from build123d import *

# Parameters (mm, degrees)
SKETCH_1_W                  = 80
SKETCH_1_H                  = 60
EXTRUDE_1_DEPTH             = 20
SKETCH_2_W                  = 72
SKETCH_2_H                  = 52
CUT_EXTRUDE_1_DEPTH         = 15
CUT_EXTRUDE_2_DEPTH         = 53.201532545
SKETCH_4_R                  = 1.6
CUT_EXTRUDE_3_DEPTH         = 53.201532545
PATTERN_LINEAR_1_COUNT      = 2
PATTERN_LINEAR_1_PITCH      = 60
PATTERN_LINEAR_1_COUNT_DIR2 = 2
PATTERN_LINEAR_1_PITCH_DIR2 = 40
FILLET_1_R                  = 5
SKETCH_5_W                  = 72
SKETCH_5_H                  = 52
CUT_EXTRUDE_4_DEPTH         = 1.5
SKETCH_6_W                  = 40
SKETCH_6_H                  = 8
CUT_EXTRUDE_7_DEPTH         = 85.118963379
SKETCH_7_W                  = 36
SKETCH_7_H                  = 6
CUT_EXTRUDE_8_DEPTH         = 85.118963379
SKETCH_8_W                  = 74
SKETCH_8_H                  = 54
CUT_EXTRUDE_9_DEPTH         = 1.5
SKETCH_9_W                  = 74
SKETCH_9_H                  = 54
CUT_EXTRUDE_10_DEPTH        = 1.5


with BuildPart() as part:
    # 草图1 → 凸台-拉伸1 (new body)
    with BuildSketch(Plane(origin=(0, 0, 0), x_dir=(1, 0, 0), z_dir=(0, 1, 0))):
        Rectangle(SKETCH_1_W, SKETCH_1_H)
    extrude(amount=EXTRUDE_1_DEPTH)

    # 草图2 → 切除-拉伸1 (cut)
    with BuildSketch(Plane(origin=(0, 20, 0), x_dir=(1, 0, 0), z_dir=(0, 1, 0))):
        Rectangle(SKETCH_2_W, SKETCH_2_H)
    extrude(amount=-CUT_EXTRUDE_1_DEPTH, mode=Mode.SUBTRACT)

    # 草图3 → 切除-拉伸2 (cut, through all)
    with BuildSketch(Plane(origin=(0, 5, 0), x_dir=(1, 0, 0), z_dir=(0, 1, 0))):
        Polygon((-24, 14), (-36, 14), (-36, -14), (-24, -14), (-24, -26), (24, -26), (24, -14), (36, -14), (36, 14), (24, 14), (24, 26), (-24, 26), align=None)
    extrude(amount=-CUT_EXTRUDE_2_DEPTH, mode=Mode.SUBTRACT)

    # 草图4 → 切除-拉伸3 (cut, through all)
    with BuildSketch(Plane(origin=(0, 5, 0), x_dir=(1, 0, 0), z_dir=(0, 1, 0))):
        with Locations(Location((-30, 20, 0), (0, 0, 270))):
            Circle(SKETCH_4_R)
    cut_extrude_3 = extrude(amount=-CUT_EXTRUDE_3_DEPTH, mode=Mode.SUBTRACT)

    # 阵列(线性)1: Cut-Extrude 3 2 × 2
    with Locations(*[(i * PATTERN_LINEAR_1_PITCH, 0, j * PATTERN_LINEAR_1_PITCH_DIR2) for i in range(PATTERN_LINEAR_1_COUNT) for j in range(PATTERN_LINEAR_1_COUNT_DIR2) if (i, j) != (0, 0)]):
        add(cut_extrude_3, mode=Mode.SUBTRACT)

    # 圆角1
    fillet_1_edges = [part.edges().sort_by_distance(p)[0] for p in [
        (-24, 2.5, -14),
        (24, 2.5, -14),
        (24, 2.5, 14),
        (-24, 2.5, 14),
    ]]
    fillet(fillet_1_edges, radius=FILLET_1_R)

    # 草图5 → 切除-拉伸4 (cut)
    with BuildSketch(Plane.XZ):
        Rectangle(SKETCH_5_W, SKETCH_5_H)
    extrude(amount=-CUT_EXTRUDE_4_DEPTH, mode=Mode.SUBTRACT)

    # 草图6 → 切除-拉伸7 (cut, through all)
    with BuildSketch(Plane(origin=(-36, 0, 0), x_dir=(0, 0, -1), z_dir=(1, 0, 0))):
        with Locations((0.5, 9)):
            Rectangle(SKETCH_6_W, SKETCH_6_H)
    extrude(amount=-CUT_EXTRUDE_7_DEPTH, mode=Mode.SUBTRACT)

    # 草图7 → 切除-拉伸8 (cut, through all)
    with BuildSketch(Plane.ZY.offset(-36)):
        with Locations((0, 11.5)):
            Rectangle(SKETCH_7_W, SKETCH_7_H)
    extrude(amount=-CUT_EXTRUDE_8_DEPTH, mode=Mode.SUBTRACT)

    # 草图8 → 切除-拉伸9 (cut)
    with BuildSketch(Plane(origin=(0, 20, 0), x_dir=(1, 0, 0), z_dir=(0, 1, 0))):
        Rectangle(SKETCH_8_W, SKETCH_8_H)
    extrude(amount=-CUT_EXTRUDE_9_DEPTH, mode=Mode.SUBTRACT)

    # 草图9 → 切除-拉伸10 (cut)
    with BuildSketch(Plane.XZ):
        Rectangle(SKETCH_9_W, SKETCH_9_H)
    extrude(amount=-CUT_EXTRUDE_10_DEPTH, mode=Mode.SUBTRACT)


solid = part.part
Work out the finished part from the listing and answer in its coordinate system (mm). A direction names the side the tool comes from. Give positions to 0.01 mm unless a question says otherwise; leave off trailing zeros. Loops run counter-clockwise (first coordinate to the right, second up) from the corner with the lowest first, then second, coordinate; pieces in that order, holes last. Notation, with made-up numbers: (38.5, -37) - (96.5, -37) arc R27 cw to (96.5, 1) - close; hole circle Ø5 at (73.5, 13.5). An arc over 180 degrees is marked (long way). Answer in a Markdown table with one row per item.
(1) Section A-A (x = 30) is taken. Give the vertices of the cut face in (y, z), and give its area (3 significant figures).
Results list:
| item | result |
|---|---|
| outline | (0, -30) - (20, -30) - (20, -27) - (18.5, -27) - (18.5, -26) - (5, -26) - (5, -21.6) - (1.5, -21.6) - (1.5, -27) - (0, -27) - close; (0, 27) - (1.5, 27) - (1.5, 21.6) - (5, 21.6) - (5, 26) - (18.5, 26) - (18.5, 27) - (20, 27) - (20, 30) - (0, 30) - close; (1.5, -18.4) - (5, -18.4) - (5, -14) - (1.5, -14) - close; (1.5, 14) - (5, 14) - (5, 18.4) - (1.5, 18.4) - close |
| area | 216 mm² |
(2) Flat-ended cylindrical pins translate along their axes: pin 1 Ø10 at (x, z) = (7.5, 19) entering from -Y; pin 2 Ø1 at (x, z) = (31.5, -20.5) entering from -Y; pin 3 Ø3.5 at (x, z) = (29.5, 21.5) entering from +Y. Find the tip coordinate at first contact, or state that the pin passes through.
Results list:
| item | result |
|---|---|
| pin 1 | passes through |
| pin 2 | stops at y = 1.5 |
| pin 3 | stops at y = 5 |
(3) Section B-B (y = 16.5) is taken. Give the vertices of the cut face in (x, z).
Results list:
| item | result |
|---|---|
| outline | (-40, -30) - (40, -30) - (40, 30) - (-40, 30) - close; hole (-36, -26) - (36, -26) - (36, 26) - (-36, 26) - close |
(4) A tool of negligible diameter and unlimited length cuts with its end or side. For faces 4 (the face through (-3, 20, 29)), 5 (the face through (36, 8, 0)), 6 (the face through (-1, 10, -30)), 7 (the face through (-38, 9, 19.5)), 8 (the face through (24, 3, 23)), from which of +Z, -Z, +X, -X, +Y, -Y can it reach the whole face along a straight path? Write none if from no direction.
Results list:
| item | result |
|---|---|
| face 4 | +Z, -Z, +X, -X, +Y |
| face 5 | +Y |
| face 6 | -Z, +X, -X, +Y, -Y |
| face 7 | -X |
| face 8 | +Y, -Y |
(5) For a pull along Z with two mould halves and no side action, classify faces 1 (the face through (-40, 14, 0)), 2 (the face through (-1, 10, 30)), 3 (the face through (38, 11, -18)) as pulls with the +Z half, pulls with the -Z half, needs draft (parallel to the pull), parting line crosses it, or undercut.
Results list:
| item | result |
|---|---|
| face 1 | needs draft |
| face 2 | pulls with the +Z half |
| face 3 | undercut |
(6) Section C-C (x = -5) is taken. Give the vertices of the cut face in (y, z), and give its area (3 significant figures).
Results list:
| item | result |
|---|---|
| outline | (0, -30) - (20, -30) - (20, -27) - (18.5, -27) - (18.5, -26) - (1.5, -26) - (1.5, -27) - (0, -27) - close; (0, 27) - (1.5, 27) - (1.5, 26) - (18.5, 26) - (18.5, 27) - (20, 27) - (20, 30) - (0, 30) - close |
| area | 154 mm² |
(7) Consider L1, parallel to X at y = 3.5, z = 20; L2, parallel to X at y = 18.75, z = -2; L3, parallel to X at y = 16.5, z = -16. Determine where each line is inside the solid, lowest interval first. Write a range as [from, to].
Results list:
| item | result |
|---|---|
| L1 | x = [-40, -31.6], [-28.4, -24], [24, 28.4], [31.6, 40] |
| L2 | x = [-40, -37], [37, 40] |
| L3 | x = [-40, -36], [36, 40] |
(8) Section D-D (y = 6.75) is taken. Give the vertices of the cut face in (x, z).
Results list:
| item | result |
|---|---|
| outline | (-40, -30) - (40, -30) - (40, 30) - (-40, 30) - (-40, 19.5) - (-36, 19.5) - (-36, 26) - (36, 26) - (36, -26) - (-36, -26) - (-36, -20.5) - (-40, -20.5) - close |
